```python
from build123d import *

# Parameters (mm, degrees)
BOSS_EXTRUDE1_DEPTH = 50
FILLET1_R           = 10
SKETCH2_W           = 6.733148768
SKETCH2_H           = 28.503663117
BOSS_EXTRUDE2_DEPTH = 6
CUT_EXTRUDE1_DEPTH  = 29


with BuildPart() as part:
    # Sketch1 → Boss-Extrude1 (new body)
    with BuildSketch(Plane(origin=(0, 0, 0), x_dir=(1, 0, 0), z_dir=(0, 1, 0))):
        with BuildLine():
            Line((0, -33.816412485), (52.662713514, 0))
            Line((52.662713514, 0), (0, 33.816412485))
            Line((0, 33.816412485), (-42.662713514, 33.816412485))
            ThreePointArc((-42.662713514, 33.816412485), (-49.733781326, 30.887480297), (-52.662713514, 23.816412485))
            Line((-52.662713514, 23.816412485), (-52.662713514, -23.816412485))
            ThreePointArc((-52.662713514, -23.816412485), (-49.733781326, -30.887480297), (-42.662713514, -33.816412485))
            Line((-42.662713514, -33.816412485), (0, -33.816412485))
        make_face()
    extrude(amount=BOSS_EXTRUDE1_DEPTH)

    # Fillet1
    fillet1_edges = [part.edges().sort_by_distance(p)[0] for p in [
        (-49.733781326, 50, -30.887480297),
        (-52.662713514, 50, 0),
        (-49.733781326, 50, 30.887480297),
        (-21.331356757, 50, 33.816412485),
        (-21.331356757, 50, -33.816412485),
    ]]
    fillet(fillet1_edges, radius=FILLET1_R)

    # Sketch2 → Boss-Extrude2 (add)
    with BuildSketch(Plane.XY.offset(33.816412485)):
        with Locations((-34.339058715, 18.322960806)):
            Rectangle(SKETCH2_W, SKETCH2_H)
    extrude(amount=BOSS_EXTRUDE2_DEPTH)

    # Sketch3 → Cut-Extrude1 (cut)
    with BuildSketch(Plane(origin=(0, 4.071129247, 0), x_dir=(-1, 0, 0), z_dir=(0, -1, 0))):
        Polygon((30.972484331, -33.816412485), (36.246784199, -39.816412485), (30.972484331, -39.816412485), align=None)
    extrude(amount=-CUT_EXTRUDE1_DEPTH, mode=Mode.SUBTRACT)


solid = part.part
```
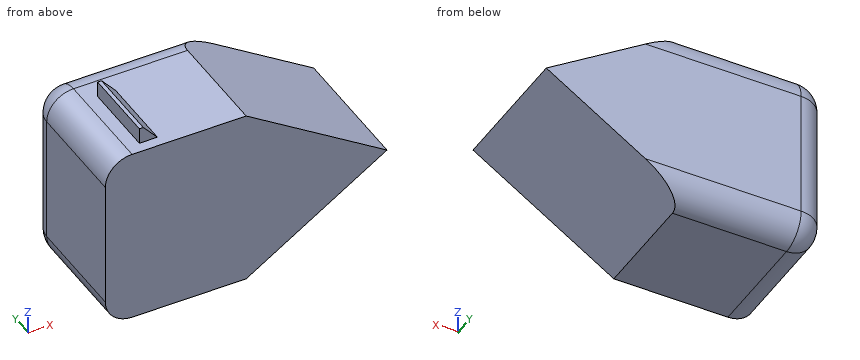
The model under review builds one solid part; all positions refer to its coordinate system, in mm. Coordinates: 2 decimals unless noted, no trailing zeros. Write each loop counter-clockwise with the first axis right and the second up, starting at its lowest first coordinate (ties: lowest second). Pieces come first, ordered by that corner, then holes.
1) To check wall thickness, follow probe 1 along Z at (x, y) = (-27, 39); probe 2 along Y at (x, z) = (-19, -26); probe 3 along X at (y, z) = (36.5, -19). State the ranges of each line that lie inside material, in increasing order.
2) We need section A-A on y = 28.5. State the section outline as (x, z) points, then the cut area to 3 significant figures.
3) We need section C-C on z = 4. State the section outline as (x, y) points, then the cut area to 3 significant figures.
4) We need section D-D on z = 28.5. State the section outline as (x, y) points, then the cut area to 3 significant figures.
5) Clearance check with flat-ended pins moving along their axes: pin 1 Ø1.5 at (y, z) = (22.5, 11.5) entering from +X; pin 2 Ø1.8 at (x, z) = (-34, 36.5) entering from +Y; pin 3 Ø5 at (x, z) = (-32.5, 38.5) entering from -Y. State where each tip first meets the part, or that it passes through.
6) We need section B-B on x = -21. State the section outline as (y, z) points.
Answer list:
1. probe 1: z = -33.82 to 33.82
1. probe 2: y = 0 to 49.76
1. probe 3: x = -52.66 to 23.07
2. outline: (-52.66, -23.82) arc R10 ccw to (-42.66, -33.82) - (0, -33.82) - (52.66, 0) - (0, 33.82) - (-30.97, 33.82) - (-36.25, 39.82) - (-37.71, 39.82) - (-37.71, 33.82) - (-42.66, 33.82) arc R10 ccw to (-52.66, 23.82) - close
2. area: 5,320 mm2
3. outline: (-52.66, 0) - (46.43, 0) - (46.43, 50) - (-42.66, 50) arc R10 ccw to (-52.66, 40) - close
3. area: 4,930 mm2
4. outline: (-51.5, 0) - (8.28, 0) - (8.28, 48.84) - (-42.66, 48.84) arc R8.84 ccw to (-51.5, 40) - close
4. area: 2,900 mm2
5. pin 1: stops at x = 35.92
5. pin 2: stops at y = 32.57
5. pin 3: stops at y = 4.07
6. outline: (0, -33.82) - (40, -33.82) arc R10 ccw to (50, -23.82) - (50, 23.82) arc R10 ccw to (40, 33.82) - (0, 33.82) - close
